```python
from build123d import *

# Parameters (mm, degrees)
F0_W     = 60
F0_H     = 60
F0_W_2   = 40
F0_H_2   = 40
F1_DEPTH = 30
F2_W     = 40
F2_H     = 40
F3_DEPTH = 60.001
F4_W     = 40
F4_H     = 40
F5_DEPTH = 60.001


with BuildPart() as f1:
    # F0 (on Front) → F1 (new body, symmetric)
    with BuildSketch(Plane.XZ):
        Rectangle(F0_W, F0_H)
        Rectangle(F0_W_2, F0_H_2, mode=Mode.SUBTRACT)
    extrude(amount=F1_DEPTH, both=True)

    # F2 (on face) → F3 (cut, through all)
    with BuildSketch(Plane.YZ.offset(30)):
        Rectangle(F2_W, F2_H)
    extrude(amount=-F3_DEPTH, mode=Mode.SUBTRACT)

    # F4 (on face) → F5 (cut, through all)
    with BuildSketch(Plane.XY.offset(30)):
        Rectangle(F4_W, F4_H)
    extrude(amount=-F5_DEPTH, mode=Mode.SUBTRACT)


solid = f1.part
```
Read the model definition and answer for the solid it produces. Units are mm, in the model's axes. A direction names the side the tool comes from. Coordinates: 2 decimals unless noted, no trailing zeros. Loops run counter-clockwise (first coordinate to the right, second up) from the corner with the lowest first, then second, coordinate; pieces in that order, holes last.
(1) Consider line 1 along X through (y, z) = (24.5, 18). Determine where the line is inside the solid, lowest interval first.
Solution:
line 1: x = -30 to -20, 20 to 30
(2) The part is cut by section C-C (z = -24). Determine the outline of the cut face in (x, y), and give its area (3 significant figures).
Solution:
outline: (-30, -30) - (30, -30) - (30, 30) - (-30, 30) - close; hole (-20, -20) - (20, -20) - (20, 20) - (-20, 20) - close
area: 2,000 mm2
(3) A tool of negligible diameter and unlimited length cuts with its end or side. For faces 1 (the face through (0, -20, -25)), 2 (the face through (-20, -25, 0)), 3 (the face through (25, 20, 0)), from which of +Z, -Z, +X, -X, +Y, -Y can it reach the whole face along a straight path? Write none if from no direction.
Solution:
face 1: +Z, -Z
face 2: +Y, -Y
face 3: +X, -X
(4) The part is cut by section A-A (x = 8). Determine the outline of the cut face in (y, z), and give its area (3 significant figures).
Solution:
outline: (-30, -30) - (-20, -30) - (-20, -20) - (-30, -20) - close; (-30, 20) - (-20, 20) - (-20, 30) - (-30, 30) - close; (20, -30) - (30, -30) - (30, -20) - (20, -20) - close; (20, 20) - (30, 20) - (30, 30) - (20, 30) - close
area: 400 mm2
(5) The mould has two halves that part along X. Classify faces 4 (the face through (-20, 0, -25)), 5 (the face through (25, -20, 0)), 6 (the face through (-30, -0.4, -20.4)): released by +X, released by -X, zero draft, split by the parting line, or undercut.
Solution:
face 4: undercut
face 5: zero draft
face 6: released by -X
